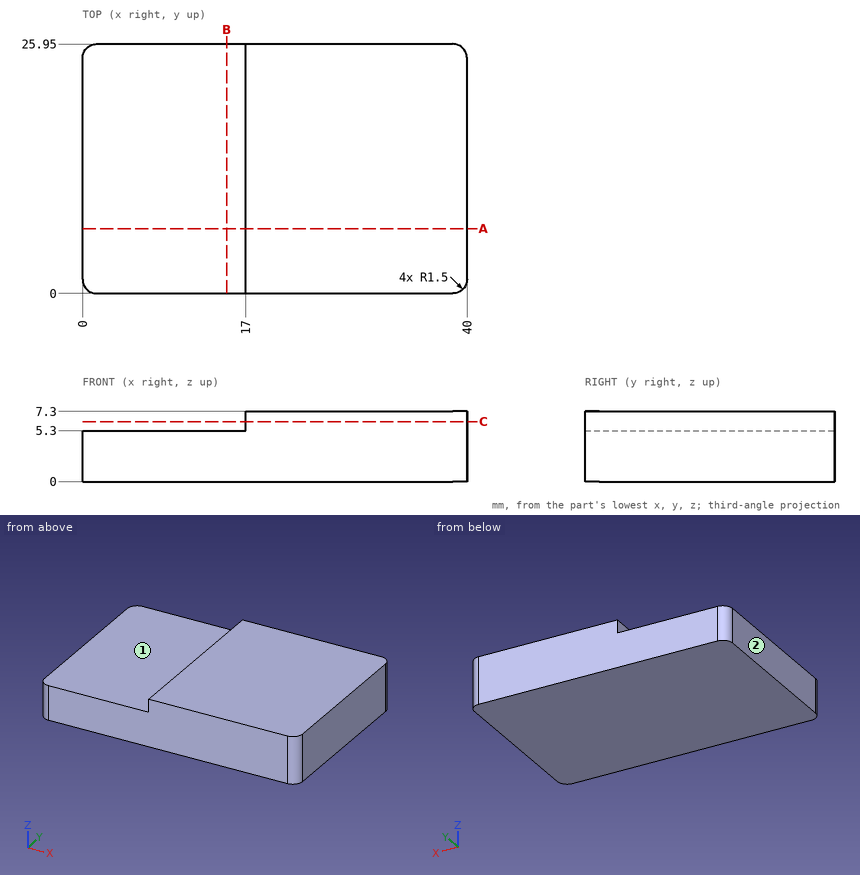
The figure shows three views and two pictorial views of one solid part (mm, origin at its lowest corner). Answer the questions. A direction names the side the tool comes from. Coordinates: 2 decimals unless noted, no trailing zeros. Loops run counter-clockwise (first coordinate to the right, second up) from the corner with the lowest first, then second, coordinate; pieces in that order, holes last. Notation, with made-up numbers: (56, 10.5) - (103, 10.5) arc R35 cw to (103, 48.5) - close; hole circle Ø4 at (82, 38.25). An arc over 180 degrees is marked (long way). Use a Markdown table: item, result. Add a question column.
1) Find the intervals of material crossed by line 1 (Z direction, x = 10.5, y = 5); line 2 (X direction, y = 18.75, z = 6), in increasing order.
2) The part is cut by section C-C, the plane z = 6.25. Give the vertices of the cut face in (x, y), and give its area (3 significant figures).
3) The part is cut by section A-A, the plane y = 6.75. Give the vertices of the cut face in (x, z), and give its area (3 significant figures).
4) For the marked faces 1 and 2, determine the directions among +Z, -Z, +X, -X, +Y, -Y from which every point of the face is accessible in a straight line to the end or side of a thin tool.
5) The part is cut by section B-B, the plane x = 15. Give the vertices of the cut face in (y, z).
6) Given pin 1 (5 mm diameter, centred on x = 9.5, y = 11.5, fed in from +Z); pin 2 (12 mm diameter, centred on x = 9, y = 4, fed in from -Z), each flat-ended and moving along its own axis, determine where each tip first touches the part or whether it passes through.
Here are the results:
| question | item | result |
|---|---|---|
| 1 | line 1 | z = 0 to 5.3 |
| 1 | line 2 | x = 17 to 40 |
| 2 | outline | (17, 0) - (38.5, 0) arc R1.5 ccw to (40, 1.5) - (40, 24.45) arc R1.5 ccw to (38.5, 25.95) - (17, 25.95) - close |
| 2 | area | 596 mm^2 |
| 3 | outline | (0, 0) - (40, 0) - (40, 7.3) - (17, 7.3) - (17, 5.3) - (0, 5.3) - close |
| 3 | area | 258 mm^2 |
| 4 | face 1 | +Z, -X, +Y, -Y |
| 4 | face 2 | +Z, -Z, -X, +Y, -Y |
| 5 | outline | (0, 0) - (25.95, 0) - (25.95, 5.3) - (0, 5.3) - close |
| 6 | pin 1 | stops at z = 5.3 |
| 6 | pin 2 | stops at z = 0 |
